Can you work these out from the model? Positions are in its coordinate system, mm. Face numbers are marked on the shaded views. Coordinates: 2 decimals unless noted, no trailing zeros. Loops run counter-clockwise (first coordinate to the right, second up) from the corner with the lowest first, then second, coordinate; pieces in that order, holes last.
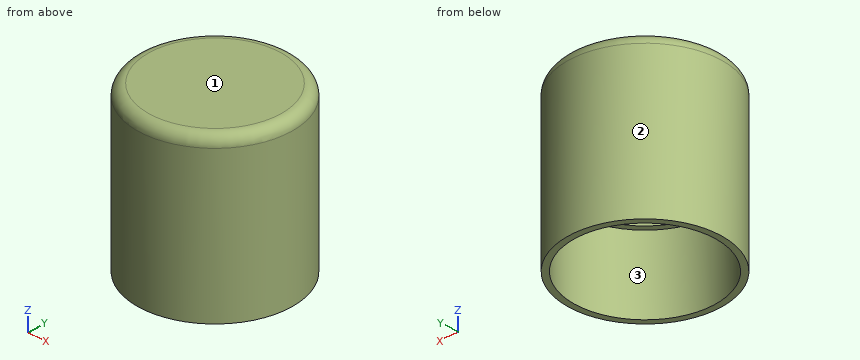
```python
from build123d import *

# Parameters (mm, degrees)
F0_R     = 50
F0_R_2   = 46
F0_R_3   = 42
F1_DEPTH = 5
F2_DEPTH = 50
F3_DEPTH = 100
F4_R     = 7


with BuildPart() as f1:
    # F0 (on Top) → F1 (new body)
    with BuildSketch(Plane.XY):
        Circle(F0_R)
        Circle(F0_R_2, mode=Mode.SUBTRACT)
        Circle(F0_R_2)
        Circle(F0_R_3, mode=Mode.SUBTRACT)
        Circle(F0_R_3)
    extrude(amount=F1_DEPTH)

    # F0 (on Top) → F2 (join)
    with BuildSketch(Plane.XY):
        Circle(F0_R_2)
        Circle(F0_R_3, mode=Mode.SUBTRACT)
    extrude(amount=-F2_DEPTH)

    # F0 (on Top) → F3 (join)
    with BuildSketch(Plane.XY):
        Circle(F0_R)
        Circle(F0_R_2, mode=Mode.SUBTRACT)
    extrude(amount=-F3_DEPTH)

    # F4
    f4_edges = [f1.edges().sort_by_distance(p)[0] for p in [
        (-50, 0, 5),
    ]]
    fillet(f4_edges, radius=F4_R)


solid = f1.part
```
Item 1: I'm going to push flat-ended pins straight in: P1, Ø8, axis at x = 28.5, y = -18, coming from the -Z side; P2, Ø12, axis at x = 15, z = -37, coming from the +Y side; P3, Ø5, axis at y = -40, z = -66.5, coming from the -X side. Where does each tip first touch, or does it pass through?
Results are:
P1: stops at z = 0
P2: stops at y = 49.18
P3: stops at x = -33.07
Item 2: We'd pull the mould along X, two halves only. Please class the marked faces 1, 2 and 3: +X half, -X half, draft (parallel to the pull), parting line (faces both ways), or undercut.
Results are:
face 1: draft
face 2: parting line
face 3: undercut
Item 3: Suppose I cut it at A-A, the plane x = 0. Please give me the cut outline in (y, z).
Results are:
outline: (-50, -100) - (-46, -100) - (-46, -50) - (-42, -50) - (-42, 0) - (42, 0) - (42, -50) - (46, -50) - (46, -100) - (50, -100) - (50, -2) arc R7 ccw to (43, 5) - (-43, 5) arc R7 ccw to (-50, -2) - close
Item 4: I need wall thicknesses on line 1 along Y through (x, z) = (0, -80); line 2 along Y through (x, z) = (0, -30.5); line 3 along Z through (x, y) = (41, -4). Which ranges of each line are inside material? Lowest first, please.
Results are:
line 1: y = -50 to -46, 46 to 50
line 2: y = -50 to -42, 42 to 50
line 3: z = 0 to 5
Item 5: Suppose I cut it at D-D, the plane z = -83. Please give me the cut outline in (x, y), plus the area to 3 significant figures.
Results are:
outline: circle Ø100 at (0, 0); hole circle Ø92 at (0, 0)
area: 1,210 mm2
Item 6: Suppose I cut it at C-C, the plane z = -3.5. Please give me the cut outline in (x, y), plus the area to 3 significant figures.
Results are:
outline: circle Ø100 at (0, 0); hole circle Ø84 at (0, 0)
area: 2,310 mm2
